from build123d import *

# Parameters (mm, degrees)
SKETCH1_W           = 99
SKETCH1_H           = 6
BOSS_EXTRUDE1_DEPTH = 2
SKETCH2_W           = 101
SKETCH2_H           = 8
BOSS_EXTRUDE3_DEPTH = 2
DRAFT1_ANGLE        = 10
SKETCH3_W           = 103
SKETCH3_H           = 10
BOSS_EXTRUDE4_DEPTH = 2
FILLET1_R           = 2


with BuildPart() as part:
    # Sketch1 → Boss-Extrude1 (new body)
    with BuildSketch(Plane(origin=(0, 0, 0), x_dir=(1, 0, 0), z_dir=(0, 1, 0))):
        Rectangle(SKETCH1_W, SKETCH1_H)
    extrude(amount=BOSS_EXTRUDE1_DEPTH)

    # Draft1
    draft1_faces = [part.faces().sort_by_distance(p)[0] for p in [
        (49.5, 1, 0),
        (0, 1, 3),
        (-49.5, 1, 0),
        (0, 1, -3),
    ]]
    draft(draft1_faces, Plane(origin=(0, 0, 0), x_dir=(0, 0, -1), z_dir=(0, -1, 0)), DRAFT1_ANGLE)



with BuildPart() as body_2:
    # Sketch2 → Boss-Extrude3 (new body)
    with BuildSketch(Plane(origin=(0, 2, 0), x_dir=(1, 0, 0), z_dir=(0, 1, 0))):
        Rectangle(SKETCH2_W, SKETCH2_H)
    extrude(amount=BOSS_EXTRUDE3_DEPTH)


with BuildPart() as part_1:
    add(part.part)

    add(body_2.part)  # Boss-Extrude4 merges body 2
    # Sketch3 → Boss-Extrude4 (add)
    with BuildSketch(Plane(origin=(0, 4, 0), x_dir=(1, 0, 0), z_dir=(0, 1, 0))):
        Rectangle(SKETCH3_W, SKETCH3_H)
    extrude(amount=-BOSS_EXTRUDE4_DEPTH)

    # Fillet1
    fillet1_edges = [part_1.edges().sort_by_distance(p)[0] for p in [
        (-51.5, 3, 5),
        (-51.5, 3, -5),
        (51.5, 3, -5),
        (51.5, 3, 5),
    ]]
    fillet(fillet1_edges, radius=FILLET1_R)


solid = part_1.part
Design review of the part built by this model. Coordinates are the model's own, in mm. Give positions to 0.01 mm unless a question says otherwise; leave off trailing zeros. Order: outer loops, then holes, each group sorted by start corner. A loop starts at its lowest first (then second) coordinate and runs counter-clockwise, first axis right, second up.
1. Add section A-A, the plane x = -37.5. State the section outline as (y, z) points, then the cut area to 3 significant figures.
Solution:
outline: (0, -3) - (2, -3.35) - (2, -5) - (4, -5) - (4, 5) - (2, 5) - (2, 3.35) - (0, 3) - close
area: 32.7 mm2
2. Add section B-B, the plane z = 0. State the section outline as (x, y) points.
Solution:
outline: (-51.5, 2) - (-49.85, 2) - (-49.5, 0) - (49.5, 0) - (49.85, 2) - (51.5, 2) - (51.5, 4) - (-51.5, 4) - close
3. Add section C-C, the plane y = 0.85. State the section outline as (x, z) points.
Solution:
outline: (-49.65, -3.15) - (49.65, -3.15) - (49.65, 3.15) - (-49.65, 3.15) - close
4. To check wall thickness, follow L1, parallel to Y at x = -11.5, z = 4.25; L2, parallel to Z at x = -45, y = 1.5; L3, parallel to Z at x = 22, y = 0.4. State the ranges of each line that lie inside material, in increasing order.
Solution:
L1: y = 2 to 4
L2: z = -3.26 to 3.26
L3: z = -3.07 to 3.07
5. For pin 1 Ø1.5 at (y, z) = (0.5, -1.5) entering from +X, flat-tipped, find the tip position at first contact; note if it passes through.
Solution:
pin 1: stops at x = 49.72
